Drawing for the job (mm, zero at the part's lowest x, y, z). A direction names the side the tool comes from. Give positions to 0.01 mm unless a question says otherwise; leave off trailing zeros. Loops run counter-clockwise (first coordinate to the right, second up) from the corner with the lowest first, then second, coordinate; pieces in that order, holes last. Notation, with made-up numbers: (79.25, 36.25) - (105.25, 36.25) arc R33 ccw to (105.25, 74.25) - close; hole circle Ø10 at (-21.75, 37). An arc over 180 degrees is marked (long way). Return JSON: item names as keys, results as strings. Group by question number.
1) Mould opens along Z. For the marked faces 1, 2 and 3 say: released by +Z, released by -Z, zero draft, split by the parting line, or undercut.
2) Drill centre lines: probe 1 along Z at (x, y) = (6.5, 4.5); probe 2 along X at (y, z) = (5.5, 7.75) (1 decimal); probe 3 along X at (y, z) = (5, 2.25) (1 decimal). Where is each one in solid material? Low to high. Write a range as from..to.
3) Slice it at D-D (x = 5.25). List the corners of the cut face in (y, z).
4) 3-axis set-ups, long thin cutter, end or side, ignore diameter. For the marked faces 4, 5, 6 and 7: which of +Z, -Z, +X, -X, +Y, -Y reach the whole face in a straight line?
5) Slice it at A-A (y = 4). List the corners of the cut face in (x, z) (1 decimal).
6) Drop flat-ended pins along their axis: pin 1 (0.6 mm diameter, centred on y = 2.5, z = 8.5, fed in from -X) (3 decimals); pin 2 (1.6 mm diameter, centred on y = 5, z = 4, fed in from -X) (3 decimals); pin 3 (4 mm diameter, centred on y = 4.5, z = 5, fed in from +X) (3 decimals). Give the stop position or say it passes through.
7) Slice it at C-C (z = 4.75). Count the separate pieces of the cut face and the enclosed holes in it, and give its area (3 significant figures).
8) Slice it at B-B (z = 8). List the corners of the cut face in (x, y) (1 decimal).
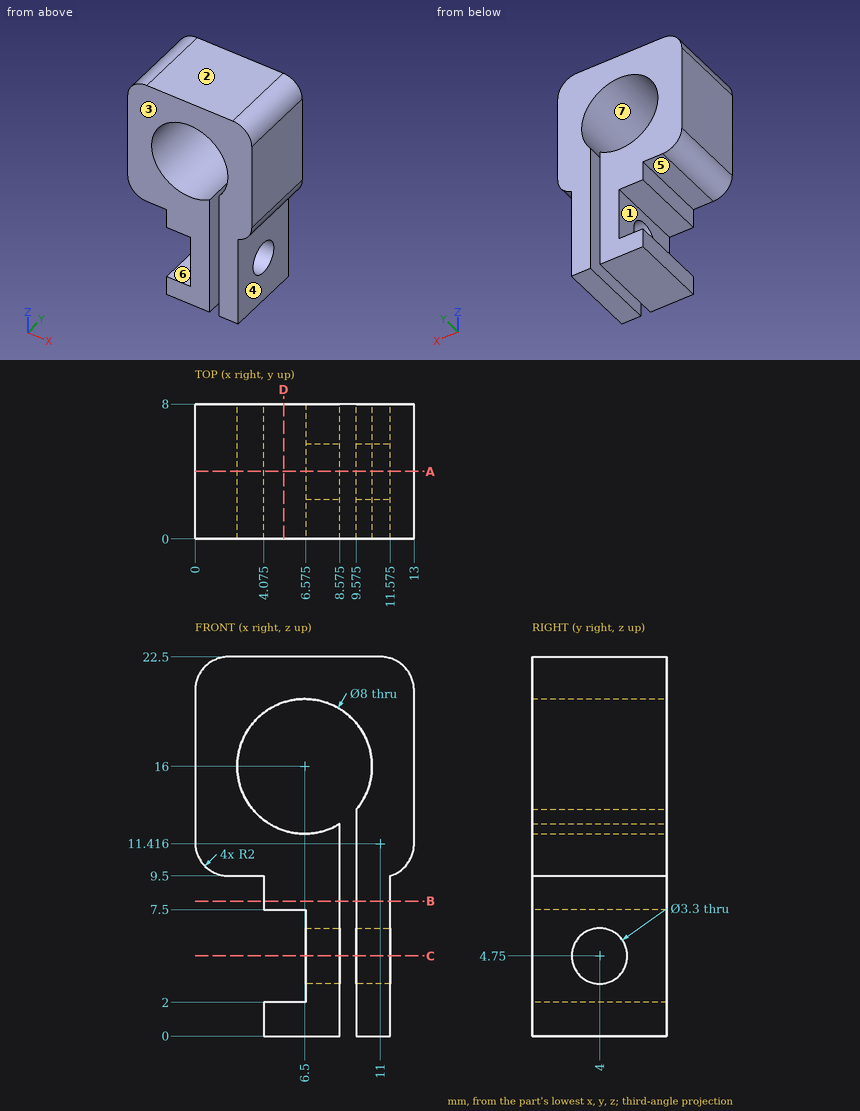
Results:
{
 "1": {"face 1": "undercut", "face 2": "released by +Z", "face 3": "zero draft"},
 "2": {"probe 1": "0..2, 7.5..12, 20..22.5", "probe 2": "4.1..8.6, 9.6..11.6", "probe 3": "6.6..8.6, 9.6..11.6"},
 "3": {"outline": "(0, 0) - (8, 0) - (8, 2) - (0, 2) - close; (0, 7.5) - (8, 7.5) - (8, 12.2) - (0, 12.2) - close; (0, 19.8) - (8, 19.8) - (8, 22.5) - (0, 22.5) - close"},
 "4": {"face 4": "-Z, +X, +Y, -Y", "face 5": "-Z, -X, +Y, -Y", "face 6": "-X, +Y, -Y", "face 7": "+Y, -Y"},
 "5": {"outline": "(0, 11.5) arc R2 ccw to (2, 9.5) - (4.1, 9.5) - (4.1, 7.5) - (6.6, 7.5) - (6.6, 6.4) - (8.6, 6.4) - (8.6, 12.6) arc R4 cw (long way) to (9.6, 13.4) - (9.6, 6.4) - (11.6, 6.4) - (11.6, 9.5) arc R2 ccw to (13, 11.4) - (13, 20.5) arc R2 ccw to (11, 22.5) - (2, 22.5) arc R2 ccw to (0, 20.5) - close; (4.1, 0) - (8.6, 0) - (8.6, 3.1) - (6.6, 3.1) - (6.6, 2) - (4.1, 2) - close; (9.6, 0) - (11.6, 0) - (11.6, 3.1) - (9.6, 3.1) - close"},
 "6": {"pin 1": "x = 4.075", "pin 2": "x = 6.575", "pin 3": "x = 11.575"},
 "7": {"separate pieces": "4", "enclosed holes": "0", "area": "18.8 mm2"},
 "8": {"outline": "(4.1, 0) - (8.6, 0) - (8.6, 8) - (4.1, 8) - close; (9.6, 0) - (11.6, 0) - (11.6, 8) - (9.6, 8) - close"}
}
